from build123d import *

# Parameters (mm, degrees)
F0_W     = 63
F0_H     = 16
F1_DEPTH = 10
F2_R     = 3
F2_R_2   = 6
F3_DEPTH = 10.001
F2_R_3   = 5.1
F4_DEPTH = 6.1
F5_R     = 1.5
F6_DEPTH = 4.1915250807
F7_R     = 5
F8_DEPTH = 5


with BuildPart() as f1:
    # F0 (on Top) → F1 (new body)
    with BuildSketch(Plane.XY):
        with Locations((31.5, 8)):
            Rectangle(F0_W, F0_H)
    extrude(amount=F1_DEPTH)

    # F2 (on face) → F3 (cut, through all)
    with BuildSketch(Plane.XY.offset(10)):
        with Locations((8, 8)):
            Circle(F2_R)
        with Locations((53, 8)):
            Circle(F2_R_2)
    extrude(amount=-F3_DEPTH, mode=Mode.SUBTRACT)

    # F2 (on face) → F4 (cut)
    with BuildSketch(Plane.XY.offset(10)):
        with Locations((8, 8)):
            Circle(F2_R_3)
        with Locations((8, 8)):
            Circle(F2_R, mode=Mode.SUBTRACT)
    extrude(amount=-F4_DEPTH, mode=Mode.SUBTRACT)

    # F5 (on face) → F6 (cut, through all)
    with BuildSketch(Plane.YZ.offset(63)):
        with Locations((8, 5)):
            Circle(F5_R)
    extrude(amount=-F6_DEPTH, mode=Mode.SUBTRACT)

    # F7 (on face) → F8 (cut)
    with BuildSketch(Plane(origin=(0, 0, 0), x_dir=(1, 0, 0), z_dir=(0, 0, -1))):
        with Locations((34, -8)):
            Circle(F7_R)
    extrude(amount=-F8_DEPTH, mode=Mode.SUBTRACT)


solid = f1.part
Model file for the job. Use its own axes, mm. A direction names the side the tool comes from. Coordinates: 2 decimals unless noted, no trailing zeros. Order: outer loops, then holes, each group sorted by start corner. A loop starts at its lowest first (then second) coordinate and runs counter-clockwise, first axis right, second up. Notation, with made-up numbers: (-36.75, 46) -> (0.25, 46) arc R18 ccw to (0.25, 72) -> close; hole circle Ø1 at (-16.75, 43). An arc over 180 degrees is marked (long way). Return JSON: item names as keys, results as strings. Group by question number.
Item 1: Saw through at D-D on x = 34. Write the cut outline in (y, z).
Item 2: Flat gauge pins, fed straight in: P1, Ø5, axis at x = 9, y = 9.5, coming from the +Z side; P2, Ø1.8, axis at y = 8, z = 5, coming from the +X side. Where does each tip first touch, or does it go through?
Item 3: Wall check: line 1 along Y through (x, z) = (59.8, 5); line 2 along Y through (x, z) = (53, 5.75); line 3 along X through (y, z) = (8.5, 8.5). Give the ranges that are in metal, low to high. Write a range as [from, to].
Item 4: Tool access for faces 5 (the cylindrical face through (10.74, 12.3, 6.99)), 6 (the cylindrical face through (47, 8, 5)), 7 (the flat face through (34, 8, 5)): list every direction of +Z, -Z, +X, -X, +Y, -Y with a clear straight run to the whole face (end or side of a thin tool).
Item 5: Saw through at B-B on y = 8. Write the cut outline in (x, z), then the cut area to 3 significant figures.
Item 6: Pull direction Y, two halves, no side cores. Call faces 1 (the cylindrical face through (60.9, 6.8, 4.1)), 2 (the flat face through (24, 8, 0)), 3 (the flat face through (31, 0, 5)), 4 (the flat face through (31, 16, 5)): pulls with the +Y half, pulls with the -Y half, needs draft (parallel to the pull), parting line crosses it, or undercut.
Item 7: Saw through at A-A on x = 53. Write the cut outline in (y, z), then the cut area to 3 significant figures.
Item 8: Saw through at C-C on z = 1. Write the cut outline in (x, y).
Values found:
{
 "1": {"outline": "(0, 0) -> (3, 0) -> (3, 5) -> (13, 5) -> (13, 0) -> (16, 0) -> (16, 10) -> (0, 10) -> close"},
 "2": {"P1": "stops at z = 3.9", "P2": "stops at x = 47.07"},
 "3": {"line 1": "y = [0, 6.5], [9.5, 16]", "line 2": "y = [0, 2], [14, 16]", "line 3": "x = [0, 2.92], [13.08, 47.02], [58.98, 63]"},
 "4": {"face 5": "+Z", "face 6": "+Z, -Z", "face 7": "-Z"},
 "5": {"outline": "(0, 0) -> (5, 0) -> (5, 3.9) -> (2.9, 3.9) -> (2.9, 10) -> (0, 10) -> close; (11, 0) -> (29, 0) -> (29, 5) -> (39, 5) -> (39, 0) -> (47, 0) -> (47, 10) -> (13.1, 10) -> (13.1, 3.9) -> (11, 3.9) -> close; (59, 0) -> (63, 0) -> (63, 3.5) -> (59, 3.5) -> close; (59, 6.5) -> (63, 6.5) -> (63, 10) -> (59, 10) -> close", "area": "362 mm2"},
 "6": {"face 1": "undercut", "face 2": "needs draft", "face 3": "pulls with the -Y half", "face 4": "pulls with the +Y half"},
 "7": {"outline": "(0, 0) -> (2, 0) -> (2, 10) -> (0, 10) -> close; (14, 0) -> (16, 0) -> (16, 10) -> (14, 10) -> close", "area": "40.0 mm2"},
 "8": {"outline": "(0, 0) -> (63, 0) -> (63, 16) -> (0, 16) -> close; hole circle Ø6 at (8, 8); hole circle Ø10 at (34, 8); hole circle Ø12 at (53, 8)"}
}
